from build123d import *

# Parameters (mm, degrees)
F0_R     = 5
F1_DEPTH = 10
F2_R     = 1.5
F3_DEPTH = 7
F4_R     = 1.5
F5_DEPTH = 5


with BuildPart() as f1:
    # F0 (on Top) → F1 (new body)
    with BuildSketch(Plane.XY):
        Circle(F0_R)
    extrude(amount=F1_DEPTH)

    # F2 (on face) → F3 (cut)
    with BuildSketch(Plane.XY.offset(10)):
        Circle(F2_R)
    extrude(amount=-F3_DEPTH, mode=Mode.SUBTRACT)

    # F4 (on face) → F5 (join)
    with BuildSketch(Plane(origin=(0, 0, 0), x_dir=(1, 0, 0), z_dir=(0, 0, -1))):
        Circle(F4_R)
    extrude(amount=F5_DEPTH)


solid = f1.part
The model under review builds one solid part; all positions refer to its coordinate system, in mm. A direction names the side the tool comes from. Round coordinates to 2 decimals unless told otherwise and drop trailing zeros. Order: outer loops, then holes, each group sorted by start corner. A loop starts at its lowest first (then second) coordinate and runs counter-clockwise, first axis right, second up. Notation, with made-up numbers: (16.25, 85.25) -> (73.25, 85.25) arc R7 cw to (73.25, 97.25) -> close; hole circle Ø8 at (80.5, -31). An arc over 180 degrees is marked (long way). Return JSON: item names as keys, results as strings.
1. Insertion check: P1, Ø5, axis at y = -3.5, z = -2, coming from the +X side; P2, Ø0.9, axis at x = 0, y = 0, coming from the +Z side; P3, Ø1.5, axis at x = 1.5, z = 1.5, coming from the -Y side. Each pin has a flat end and moves straight along its axis. Give the tip position at first contact, or say it passes through.
Answer block:
{"P1": "stops at x = 4.58", "P2": "stops at z = 3", "P3": "stops at y = -4.94"}
2. Take a section at A-A (x = 0). Write out the cut boundary in (y, z).
Answer block:
{"outline": "(-5, 0) -> (-1.5, 0) -> (-1.5, -5) -> (1.5, -5) -> (1.5, 0) -> (5, 0) -> (5, 10) -> (1.5, 10) -> (1.5, 3) -> (-1.5, 3) -> (-1.5, 10) -> (-5, 10) -> close"}
3. For L1, parallel to Y at x = 0, z = 7.75; L2, parallel to Z at x = 3.75, y = 1.25; L3, parallel to Y at x = -1, z = 5, list the stretches that pass through material, from the lowest coordinate up. Write a range as [from, to].
Answer block:
{"L1": "y = [-5, -1.5], [1.5, 5]", "L2": "z = [0, 10]", "L3": "y = [-4.9, -1.12], [1.12, 4.9]"}
4. Take a section at D-D (z = -1.5). Write out the cut boundary in (x, y), then the cut area to 3 significant figures.
Answer block:
{"outline": "circle Ø3 at (0, 0)", "area": "7.07 mm²"}
5. The part is to be moulded in two halves that separate along X. For faces 1 (the face through (-1.5, 0.07, 6.55)), 2 (the face through (-1.5, -0.07, -2.46)), 3 (the face through (-1.2, 1.2, 10)), say which applies: +X half, -X half, draft (parallel to the pull), parting line (faces both ways), or undercut.
Answer block:
{"face 1": "undercut", "face 2": "parting line", "face 3": "draft"}
6. For faces 4 (the face through (-1.08, -4.88, 4.93)), 5 (the face through (0, 0, 3)), 6 (the face through (-1.2, 1.2, 0)), list the 3-axis set-ups (+Z, -Z, +X, -X, +Y, -Y) from which the entire face can be reached by the end or side of a thin tool; tool diameter is ignored.
Answer block:
{"face 4": "+Z, -Z", "face 5": "+Z", "face 6": "-Z"}
7. Take a section at C-C (z = 4.75). Write out the cut boundary in (x, y), then the cut area to 3 significant figures.
Answer block:
{"outline": "circle Ø10 at (0, 0); hole circle Ø3 at (0, 0)", "area": "71.5 mm²"}
